from build123d import *

# Parameters (mm, degrees)
SKETCH_W  = 40
SKETCH_H  = 25
SKETCH_R  = 1.5
PAD_DEPTH = 3


with BuildPart() as part:
    # Sketch → Pad (new body)
    with BuildSketch(Plane.XY):
        with Locations((20, 12.5)):
            Rectangle(SKETCH_W, SKETCH_H)
        with Locations((31.5, 19.5)):
            Circle(SKETCH_R, mode=Mode.SUBTRACT)
        with Locations((31.5, 7)):
            Circle(SKETCH_R, mode=Mode.SUBTRACT)
        with Locations((5, 7)):
            Circle(SKETCH_R, mode=Mode.SUBTRACT)
    pad = extrude(amount=PAD_DEPTH)

    # Mirrored: Pad across Sketch V_Axis
    add(pad.mirror(Plane(origin=(0, 0, 0), x_dir=(0, 0, 1), z_dir=(1, 0, 0))))


solid = part.part
Part model, mm, in its own coordinate system. Round coordinates to 2 decimals unless told otherwise and drop trailing zeros. Loops run counter-clockwise (first coordinate to the right, second up) from the corner with the lowest first, then second, coordinate; pieces in that order, holes last. Notation, with made-up numbers: (78, 83) - (103, 83) arc R21 cw to (103, 116) - close; hole circle Ø1 at (-30, -22.5). An arc over 180 degrees is marked (long way). Answer as a JSON object with one key per item and string values.
Item 1: Pull direction X, two halves, no side cores. Call faces 1 (the face through (-40, 12, 1)), 2 (the face through (30, 7, 1)), 3 (the face through (1, 0, 1)): pulls with the +X half, pulls with the -X half, needs draft (parallel to the pull), parting line crosses it, or undercut.
Output:
{"face 1": "pulls with the -X half", "face 2": "undercut", "face 3": "needs draft"}
Item 2: Band-saw the part on D-D on y = 19.5. List the corners of the cut face in (x, z).
Output:
{"outline": "(-40, 0) - (-33, 0) - (-33, 3) - (-40, 3) - close; (-30, 0) - (30, 0) - (30, 3) - (-30, 3) - close; (33, 0) - (40, 0) - (40, 3) - (33, 3) - close"}
Item 3: Pin check, flat tip, straight feed: pin 1 (2.5 mm diameter, centred on x = -31.5, y = 7, fed in from -Z). Stop position of the tip, or through.
Output:
{"pin 1": "through"}
Item 4: Band-saw the part on A-A on y = 7. List the corners of the cut face in (x, z), plus the area to 3 significant figures.
Output:
{"outline": "(-40, 0) - (-33, 0) - (-33, 3) - (-40, 3) - close; (-30, 0) - (-6.5, 0) - (-6.5, 3) - (-30, 3) - close; (-3.5, 0) - (3.5, 0) - (3.5, 3) - (-3.5, 3) - close; (6.5, 0) - (30, 0) - (30, 3) - (6.5, 3) - close; (33, 0) - (40, 0) - (40, 3) - (33, 3) - close", "area": "204 mm2"}
Item 5: Band-saw the part on B-B on x = -5. List the corners of the cut face in (y, z).
Output:
{"outline": "(0, 0) - (5.5, 0) - (5.5, 3) - (0, 3) - close; (8.5, 0) - (25, 0) - (25, 3) - (8.5, 3) - close"}
Item 6: Wall check: L1, parallel to Y at x = -31.5, z = 2.35; L2, parallel to Y at x = -5, z = 0.9; L3, parallel to Y at x = 4.5, z = 2.25. Give the ranges that are in metal, low to high.
Output:
{"L1": "0 to 5.5, 8.5 to 18, 21 to 25", "L2": "0 to 5.5, 8.5 to 25", "L3": "0 to 5.59, 8.41 to 25"}
Item 7: Band-saw the part on C-C on z = 1. List the corners of the cut face in (x, y), plus the area to 3 significant figures.
Output:
{"outline": "(-40, 0) - (40, 0) - (40, 25) - (-40, 25) - close; hole circle Ø3 at (-31.5, 7); hole circle Ø3 at (-31.5, 19.5); hole circle Ø3 at (-5, 7); hole circle Ø3 at (5, 7); hole circle Ø3 at (31.5, 7); hole circle Ø3 at (31.5, 19.5)", "area": "1,960 mm2"}
